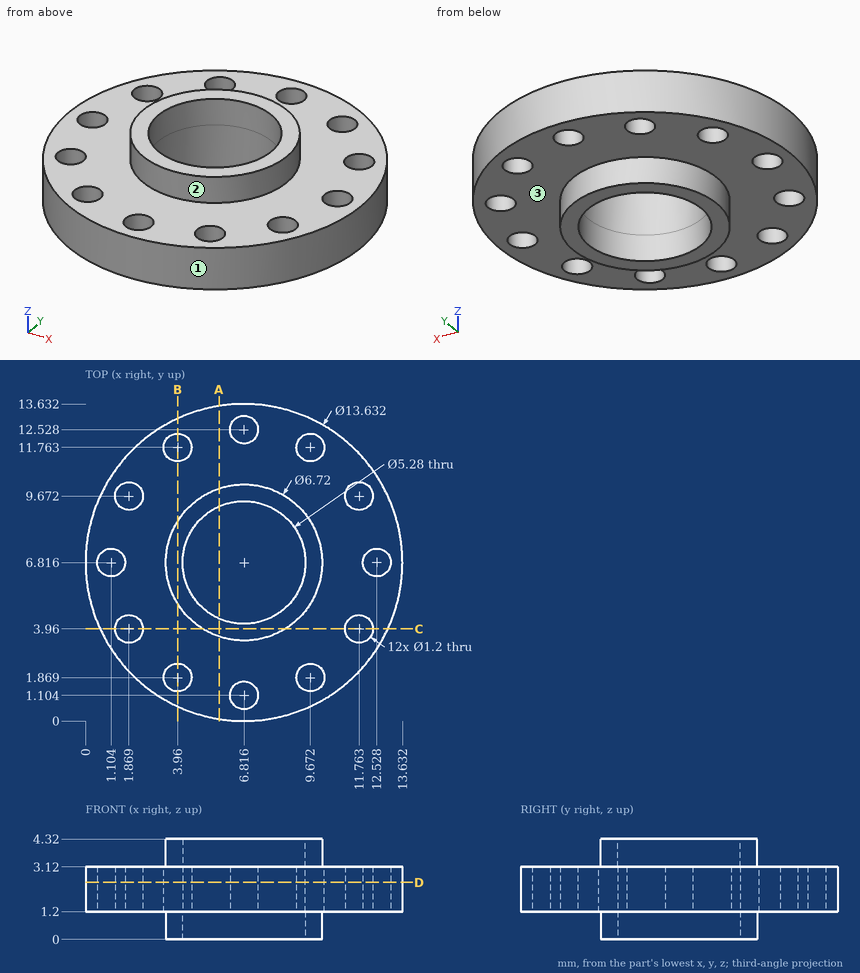
For this review, use the dimensioned drawing (mm, ordinates from the lowest corner) and the shaded views. A direction names the side the tool comes from. Give positions to 0.01 mm unless a question says otherwise; leave off trailing zeros. Write each loop counter-clockwise with the first axis right and the second up, starting at its lowest first coordinate (ties: lowest second). Pieces come first, ordered by that corner, then holes. Notation, with made-up numbers: M 57,-18 L 74,-18 A19 cw 74,7 Z; hole C 2,7.25 d2. An arc over 180 degrees is marked long. Write item = value, one per line. Start each with the question number.
Q1. Clearance check with flat-ended pins moving along their axes: pin 1 (1 mm diameter, centred on x = 6.816, y = 1.104, fed in from -Z); pin 2 (3 mm diameter, centred on x = 11.5, y = 2.5, fed in from -Z). State where each tip first meets the part, or that it passes through.
Q2. We need section D-D (z = 2.45). Give the number of separate pieces and of enclosed holes in the cut face.
Q3. Machinability: for the marked faces 1, 2 and 3, which of the approach directions +Z, -Z, +X, -X, +Y, -Y give a long, thin tool a straight path to every point of the face, cutting with its end or side? Answer none if there is none.
Q4. We need section A-A (x = 5.75). State the section outline as (y, z) points.
Q5. For line 1 (X direction, y = 7.25, z = 2.65) (1 decimal); line 2 (X direction, y = 9.75, z = 3) (1 decimal); line 3 (Y direction, x = 2.25, z = 2.3) (1 decimal), list the stretches that pass through material, from the lowest coordinate up.
Q6. We need section B-B (x = 3.96). State the section outline as (y, z) points (1 decimal).
Result set:
q1.pin_1 = through
q1.pin_2 = 1.2
q2.separate_pieces = 1
q2.enclosed_holes = 13
q3.face_1 = +Z, -Z
q3.face_2 = +Z
q3.face_3 = -Z
q4.outline = M 0.08,1.2 L 3.63,1.2 L 3.63,0 L 4.4,0 L 4.4,4.32 L 3.63,4.32 L 3.63,3.12 L 0.08,3.12 Z; M 9.23,0 L 10,0 L 10,1.2 L 13.55,1.2 L 13.55,3.12 L 10,3.12 L 10,4.32 L 9.23,4.32 Z
q5.line_1 = 0 to 0.7, 1.5 to 4.2, 9.4 to 12.1, 12.9 to 13.6
q5.line_2 = 0.7 to 1.3, 2.5 to 11.2, 12.4 to 13
q5.line_3 = 1.8 to 3.5, 4.4 to 9.2, 10.1 to 11.9
q6.outline = M 0.6,1.2 L 1.3,1.2 L 1.3,3.1 L 0.6,3.1 Z; M 2.5,1.2 L 5,1.2 L 5,0 L 8.6,0 L 8.6,1.2 L 11.2,1.2 L 11.2,3.1 L 8.6,3.1 L 8.6,4.3 L 5,4.3 L 5,3.1 L 2.5,3.1 Z; M 12.4,1.2 L 13,1.2 L 13,3.1 L 12.4,3.1 Z
